from build123d import *

# Parameters (mm, degrees)
F0_W     = 32
F0_H     = 45
F0_R     = 6.5
F1_DEPTH = 13
F2_DEPTH = 5
F3_R     = 8
F4_DEPTH = 13


with BuildPart() as f1:
    # F0 (on Top) → F1 (new body)
    with BuildSketch(Plane.XY):
        with Locations((0, 41.5)):
            Rectangle(F0_W, F0_H)
        with BuildLine():
            Line((-16, 19), (-16, 0))
            ThreePointArc((-16, 0), (0, -16), (16, 0))
            Line((16, 0), (16, 19))
            Line((16, 19), (-16, 19))
        make_face()
        Circle(F0_R, mode=Mode.SUBTRACT)
        with BuildLine():
            Line((-16, 83), (-16, 64))
            Line((-16, 64), (16, 64))
            Line((16, 64), (16, 83))
            ThreePointArc((16, 83), (0, 99), (-16, 83))
        make_face()
        with Locations((0, 83)):
            Circle(F0_R, mode=Mode.SUBTRACT)
    extrude(amount=F1_DEPTH)

    # F0 (on Top) → F2 (join)
    with BuildSketch(Plane.XY):
        with Locations((0, 41.5)):
            Rectangle(F0_W, F0_H)
    extrude(amount=-F2_DEPTH)

    # F3 (on face) → F4 (join)
    with BuildSketch(Plane.YZ.offset(16)):
        with BuildLine():
            Line((57.5, 13), (57.5, 27))
            ThreePointArc((57.5, 27), (41.5, 43), (25.5, 27))
            Line((25.5, 27), (25.5, 13))
            Line((25.5, 13), (57.5, 13))
        make_face()
        with Locations((41.5, 27)):
            Circle(F3_R, mode=Mode.SUBTRACT)
    extrude(amount=-F4_DEPTH)


solid = f1.part
Part model, mm, in its own coordinate system. A direction names the side the tool comes from. Give positions to 0.01 mm unless a question says otherwise; leave off trailing zeros. Order: outer loops, then holes, each group sorted by start corner. A loop starts at its lowest first (then second) coordinate and runs counter-clockwise, first axis right, second up. Notation, with made-up numbers: (72, 84.5) -> (131, 84.5) arc R25 ccw to (131, 98.5) -> close; hole circle Ø6 at (-36.5, 12.25). An arc over 180 degrees is marked (long way). Use one line per item in the form item = value.
(1) Pull direction X, two halves, no side cores. Call faces 4 (the face through (0, 42, -5)), 5 (the face through (-5.158, -3.955, 6.409)), 6 (the face through (16, 41, 13)): +X half, -X half, draft (parallel to the pull), parting line (faces both ways), or undercut.
Solution:
face_4 = draft
face_5 = undercut
face_6 = +X half
(2) Drill centre lines: line 1 (Y direction, x = 0, z = 7.75); line 2 (Z direction, x = 11, y = 41); line 3 (Y direction, x = 1, z = 6.5). Where is each one in solid material? Low to high. Write a range as from..to.
Solution:
line_1 = -16..-6.5, 6.5..76.5, 89.5..99
line_2 = -5..19.02, 34.98..42.99
line_3 = -15.97..-6.42, 6.42..76.58, 89.42..98.97
(3) Tool access for faces 1 (the face through (10, 57.5, 20)), 2 (the face through (0, 64, -2)), 3 (the face through (3, 6, 0)): list every direction of +Z, -Z, +X, -X, +Y, -Y with a clear straight run to the whole face (end or side of a thin tool).
Solution:
face_1 = +Z, +X, -X, +Y
face_2 = -Z, +X, -X, +Y
face_3 = -Z, +X, -X, -Y
(4) Saw through at A-A (y = 41.5). Write the cut outline in (x, z), then the cut area to 3 significant figures.
Solution:
outline = (-16, -5) -> (16, -5) -> (16, 19) -> (3, 19) -> (3, 13) -> (-16, 13) -> close; (3, 35) -> (16, 35) -> (16, 43) -> (3, 43) -> close
area = 758 mm²
(5) Saw through at B-B (x = 0). Write the cut outline in (y, z), then the cut area to 3 significant figures.
Solution:
outline = (-16, 0) -> (-6.5, 0) -> (-6.5, 13) -> (-16, 13) -> close; (6.5, 0) -> (19, 0) -> (19, -5) -> (64, -5) -> (64, 0) -> (76.5, 0) -> (76.5, 13) -> (6.5, 13) -> close; (89.5, 0) -> (99, 0) -> (99, 13) -> (89.5, 13) -> close
area = 1,380 mm²
(6) Saw through at D-D (x = -11.5). Write the cut outline in (y, z), then the cut area to 3 significant figures.
Solution:
outline = (-11.12, 0) -> (19, 0) -> (19, -5) -> (64, -5) -> (64, 0) -> (94.12, 0) -> (94.12, 13) -> (-11.12, 13) -> close
area = 1,590 mm²
(7) Flat gauge pins, fed straight in: P1, Ø1, axis at x = 5, y = 11, coming from the -Z side; P2, Ø24, axis at y = 33.5, z = 25.5, coming from the -X side; P3, Ø8, axis at x = 4.5, z = 29.5, coming from the -Y side; P4, Ø10.5, axis at x = 0, y = 83, coming from the -Z side. Where does each tip first touch, or does it go through?
Solution:
P1 = 0
P2 = 3
P3 = 25.5
P4 = through
(8) Saw through at C-C (z = 25.5). Write the cut outline in (x, y).
Solution:
outline = (3, 25.5) -> (16, 25.5) -> (16, 33.64) -> (3, 33.64) -> close; (3, 49.36) -> (16, 49.36) -> (16, 57.5) -> (3, 57.5) -> close
